Build history of the part. All positions in model axes, mm. A direction names the side the tool comes from. Give positions to 0.01 mm unless a question says otherwise; leave off trailing zeros. Loops run counter-clockwise (first coordinate to the right, second up) from the corner with the lowest first, then second, coordinate; pieces in that order, holes last. Notation, with made-up numbers: (32.25, -32) -> (88.25, -32) arc R21 cw to (88.25, -5) -> close; hole circle Ø5 at (71, 46.5). An arc over 180 degrees is marked (long way). Answer as a JSON object with one key per item and string values. Group by question number.
Q1. Two-plate mould, pull along Y, no slides. Class faces 1 (the cylindrical face through (-2.018, -15.368, -31.035)), 2 (the flat face through (-41, 10, -25)), 3 (the cylindrical face through (-68.669, 19.218, -29.19)): pulls with the +Y half, pulls with the -Y half, needs draft (parallel to the pull), parting line crosses it, or undercut.
Q2. Band-saw the part on B-B, the plane z = -22.5. Write the cut outline in (x, y), plus the area to 3 significant figures.
Q3. Band-saw the part on A-A, the plane y = 0. Write the cut outline in (x, z), plus the area to 3 significant figures.
Q4. Band-saw the part on D-D, the plane y = 30. Write the cut outline in (x, z), plus the area to 3 significant figures.
Q5. Drop flat-ended pins along their axis: pin 1 (3 mm diameter, centred on x = -20, y = 9, fed in from +Z); pin 2 (8 mm diameter, centred on y = 12.5, z = -20, fed in from -X); pin 3 (5 mm diameter, centred on x = -23, z = -8, fed in from -Y); pin 4 (5 mm diameter, centred on x = -57, z = -25.5, fed in from -Y). Give the stop position or say it passes through.
Q6. Band-saw the part on C-C, the plane x = -28.5. Write the cut outline in (y, z), plus the area to 3 significant figures.
Q7. Tool access for faces 4 (the flat face through (4, 22, -20)), 5 (the flat face through (-5.766, 21.186, -9.86)), 6 (the flat face through (-36, -16, -30)): list every direction of +Z, -Z, +X, -X, +Y, -Y with a clear straight run to the whole face (end or side of a thin tool).
Q8. Wall check: probe 1 along Y at (x, z) = (-65, -29); probe 2 along Y at (x, z) = (-68.5, -26); probe 3 along Y at (x, z) = (0, -8). Give the ranges that are in metal, low to high. Write a range as from..to.
from build123d import *

# Parameters (mm, degrees)
CUT_EXTRUDE1_DEPTH  = 20
CIRPATTERN1_COUNT   = 18
BOSS_EXTRUDE1_START = -8.5
SKETCH3_R           = 4.5
BOSS_EXTRUDE1_DEPTH = 8.5
CUT_EXTRUDE2_START  = -6
CUT_EXTRUDE2_DEPTH  = 6


with BuildPart() as part:
    # Sketch1 → Revolve2 (revolve)
    with BuildSketch(Plane(origin=(0, 0, 0), x_dir=(1, 0, 0), z_dir=(0, 1, 0)), mode=Mode.PRIVATE) as revolve2_sk:
        Polygon((-25, 0), (-14, 0), (-14, 28.5), (-15.5, 28.5), (-15.5, 33.5), (-20, 33.5), (-20, 25), (-25, 25), align=None)
    revolve(revolve2_sk.sketch.rotate(Axis((0, 0, 0), (0, 0, -1)), 180), axis=Axis((0, 0, 0), (0, 0, -1)))

    # Sketch2 → Cut-Extrude1 (cut)
    with BuildSketch(Plane.XY):
        with BuildLine():
            Line((18.894443628, 2), (24.919871589, 2))
            ThreePointArc((24.919871589, 2), (25, 0), (24.919871589, -2))
            Line((24.919871589, -2), (18.894443628, -2))
            ThreePointArc((18.894443628, -2), (19, 0), (18.894443628, 2))
        make_face()
    cut_extrude1 = extrude(amount=-CUT_EXTRUDE1_DEPTH, mode=Mode.SUBTRACT)

    # CirPattern1: Cut-Extrude1 ×18 about axis
    cirpattern1_axis = Axis((0, 0, 0), (0, 0, 1))
    for i in range(1, CIRPATTERN1_COUNT):
        add(cut_extrude1.rotate(cirpattern1_axis, i * 360 / CIRPATTERN1_COUNT), mode=Mode.SUBTRACT)

    # Sketch3 → Boss-Extrude1 (add)
    with BuildSketch(Plane(origin=(0, 0, -33.5), x_dir=(-1, 0, 0), z_dir=(0, 0, -1)).offset(BOSS_EXTRUDE1_START)):
        with BuildLine():
            Line((0, -20), (65, -20))
            ThreePointArc((65, -20), (71.363961031, -17.363961031), (74, -11))
            Line((74, -11), (74, 11))
            ThreePointArc((74, 11), (68.53379766, 19.277214151), (58.775050201, 17.5))
            Line((58.775050201, 17.5), (43.5, 17.5))
            Line((43.5, 17.5), (43.5, 40))
            Line((43.5, 40), (18.595132548, 37.821106431))
            Line((18.595132548, 37.821106431), (5.563850354, 19.210506741))
            ThreePointArc((5.563850354, 19.210506741), (19.801643048, -2.809792268), (0, -20))
        make_face()
        with Locations((65, 11)):
            Circle(SKETCH3_R, mode=Mode.SUBTRACT)
        with Locations((65, -11)):
            Circle(SKETCH3_R, mode=Mode.SUBTRACT)
    extrude(amount=BOSS_EXTRUDE1_DEPTH)

    # Sketch6 → Cut-Extrude2 (cut)
    with BuildSketch(Plane(origin=(0, 0, -33.5), x_dir=(-1, 0, 0), z_dir=(0, 0, -1)).offset(CUT_EXTRUDE2_START)):
        with BuildLine():
            Line((20.784609691, -16), (52.038518603, -16))
            ThreePointArc((52.038518603, -16), (54.973716146, -14.717464882), (56.026666725, -11.692307692))
            ThreePointArc((56.026666725, -11.692307692), (58.395805529, -4.885704016), (65, -2))
            Line((65, -2), (70, -2))
            Line((70, -2), (70, 2))
            Line((70, 2), (65, 2))
            ThreePointArc((65, 2), (59.014440454, 4.278908056), (56.06011199, 9.961538462))
            ThreePointArc((56.06011199, 9.961538462), (54.747077117, 12.487151975), (52.08682843, 13.5))
            Line((52.08682843, 13.5), (42.938553963, 13.5))
            Line((42.938553963, 13.5), (22.520523512, 6.068444673))
            ThreePointArc((22.520523512, 6.068444673), (20.505273991, 4.44346834), (19.907170071, 1.924728492))
            ThreePointArc((19.907170071, 1.924728492), (19.545454521, -4.239717862), (17.320508076, -10))
            ThreePointArc((17.320508076, -10), (17.320508076, -14), (20.784609691, -16))
        make_face()
        with BuildLine():
            Line((23.79689183, 38.276201399), (11.721526755, 21.030792837))
            ThreePointArc((11.721526755, 21.030792837), (11.038650101, 18.16861398), (12.498445777, 15.613739243))
            ThreePointArc((12.498445777, 15.613739243), (14.650735805, 13.614548849), (16.486968638, 11.3216547))
            ThreePointArc((16.486968638, 11.3216547), (18.564157588, 9.776641825), (21.152442938, 9.827215157))
            Line((21.152442938, 9.827215157), (36.868080573, 15.547239468))
            ThreePointArc((36.868080573, 15.547239468), (38.776608177, 17.011704206), (39.5, 19.306009951))
            Line((39.5, 19.306009951), (39.5, 39.650045346))
            Line((39.5, 39.650045346), (23.79689183, 38.276201399))
        make_face()
    extrude(amount=CUT_EXTRUDE2_DEPTH, mode=Mode.SUBTRACT)


solid = part.part
Worked answers:
{
 "1": {"face 1": "undercut", "face 2": "needs draft", "face 3": "pulls with the +Y half"},
 "2": {"outline": "circle Ø50 at (0, 0); hole circle Ø28 at (0, 0)", "area": "1,350 mm2"},
 "3": {"outline": "(-74, -33.5) -> (-70, -33.5) -> (-70, -27.5) -> (-20, -27.5) -> (-20, -33.5) -> (-15.5, -33.5) -> (-15.5, -28.5) -> (-14, -28.5) -> (-14, 0) -> (-19, 0) -> (-19, -20) -> (-25, -20) -> (-25, -25) -> (-74, -25) -> close; (14, -28.5) -> (15.5, -28.5) -> (15.5, -33.5) -> (20, -33.5) -> (20, -25) -> (25, -25) -> (25, -20) -> (19, -20) -> (19, 0) -> (14, 0) -> close", "area": "556 mm2"},
 "4": {"outline": "(-43.5, -33.5) -> (-39.5, -33.5) -> (-39.5, -27.5) -> (-18, -27.5) -> (-18, -33.5) -> (-13.12, -33.5) -> (-13.12, -25) -> (-43.5, -25) -> close", "area": "129 mm2"},
 "5": {"pin 1": "z = 0", "pin 2": "x = -23.51", "pin 3": "y = -14.31", "pin 4": "y = -20"},
 "6": {"outline": "(-20, -33.5) -> (-16, -33.5) -> (-16, -27.5) -> (8.24, -27.5) -> (8.24, -33.5) -> (12.5, -33.5) -> (12.5, -27.5) -> (38.69, -27.5) -> (38.69, -25) -> (-20, -25) -> close", "area": "196 mm2"},
 "7": {"face 4": "+Z", "face 5": "+Z, +Y", "face 6": "-Z"},
 "8": {"probe 1": "-20..-15.5, -6.5..-2, 2..6.5, 15.5..20", "probe 2": "-19.29..-13.83, -8.17..8.17, 13.83..19.29", "probe 3": "-25..-14, 14..25"}
}
